Work out the finished part from the listing and answer in its coordinate system (mm). Face numbers are marked on the shaded views. A direction names the side the tool comes from. Coordinates: 2 decimals unless noted, no trailing zeros. Write each loop counter-clockwise with the first axis right and the second up, starting at its lowest first coordinate (ties: lowest second). Pieces come first, ordered by that corner, then holes. Notation, with made-up numbers: (-2.75, 16.5) - (24.25, 16.5) arc R13 cw to (24.25, 33.5) - close; hole circle Ø5 at (-3.5, -25). An arc over 180 degrees is marked (long way). One line per item, written item: value.
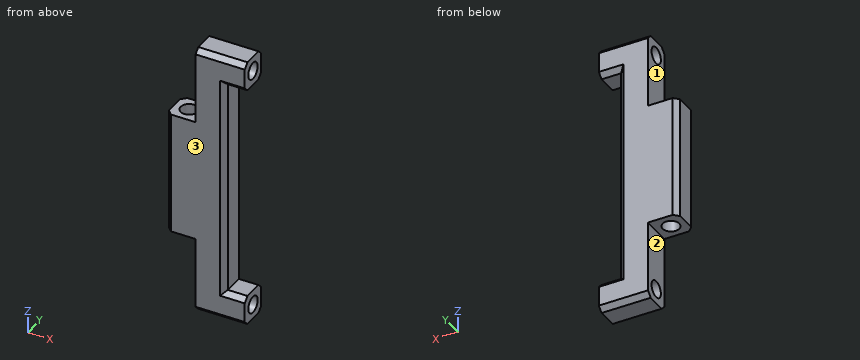
Autodesk Inventor part; units mm, degrees
ref_plane "YZ Plane" through (0, 0, 0) normal (1, 0, 0) x (0, 1, 0)
ref_plane "XZ Plane" through (0, 0, 0) normal (0, 1, 0) x (-1, 0, 0)
ref_plane "XY Plane" through (0, 0, 0) normal (0, 0, 1) x (1, 0, 0)
sketch "Sketch1" plane through (0, 0, 0) normal (0, 1, 0) x (-1, 0, 0)
  line L0 (0, 0) -> (0, -6)
  line L1 (0, -6) -> (4, -6)
  line L2 (4, -6) -> (4, -50)
  line L3 (4, -50) -> (0, -50)
  line L4 (0, -50) -> (0, -56)
  line L5 (0, -56) -> (10, -56)
  line L6 (0, 0) -> (10, 0)
  line L7 (10, 0) -> (10, -15.5)
  line L8 (10, -15.5) -> (16, -15.5)
  line L9 (16, -40.5) -> (10, -40.5)
  line L10 (10, -40.5) -> (10, -56)
  line L11 (16, -15.5) -> (16, -40.5)
  point P0 (0, -3)
  point P1 (0, -53)
  dimension "d0" = 25
  dimension "d1" = 6
  dimension "d2" = 50
  dimension "d3" = 6
  dimension "d4" = 4
  dimension "d17" = 6
extrude "Extrusion1" add sketch "Sketch1" along normal blind 6
sketch "Sketch2" plane through (0, 0, 0) normal (1, 0, 0) x (0, 0, -1)
  line L0 (15.5, 6) -> (0, 6)
  line L1 (6, 0) -> (50, 0)
  line L2 (0, 6) -> (6, 0) construction
  line L3 (50, 0) -> (56, 0)
  line L4 (50, 0) -> (56, 6) construction
  circle A0 centre (3, 3) radius 1.7
  circle A1 centre (53, 3) radius 1.7
  point P0 (0, 0)
  dimension "d8" = 3.4
extrude "Extrusion2" cut sketch "Sketch2" against normal through all
sketch "Sketch3" plane through (-16, 0, -15.5) normal (0, 0, 1) x (1, 0, 0)
  line L0 (16, 0) -> (6, 0)
  line L1 (0, 6) -> (6, 0) construction
  circle A0 centre (3, 3) radius 1.7
  dimension "d11" = 3.4
extrude "Extrusion3" cut sketch "Sketch3" against normal through all
chamfer "Chamfer1" distance 1 angle 45 12 edges at (-5, 6, 0) (-5, 0, 0) (-16, 6, -28) (-16, 0, -28) (-2, 6, -50) (-5, 6, -56) (-5, 0, -56) (-2, 0, -50) (-4, 6, -28) (-4, 0, -28) (-2, 6, -6) (-2, 0, -6)
equation "\"d3\" = d1"
equation "\"d6\" = d1"
properties part number "camadapter"
Item 1: Section A-A, the plane z = -3 is taken. Determine the outline of the cut face in (x, y), then the cut area to 3 significant figures.
Evaluation:
outline: (-10, 0) - (0, 0) - (0, 1.3) - (-10, 1.3) - close; (-10, 4.7) - (0, 4.7) - (0, 6) - (-10, 6) - close
area: 26.0 mm2
Item 2: Which of the six approach directions +Z, -Z, +X, -X, +Y, -Y give full straight-line access (tool end or side, diameter ignored) to the marked faces 1, 2 and 3?
Evaluation:
face 1: +Z, -X, +Y, -Y
face 2: -Z, -X, +Y, -Y
face 3: +Z, -Z, +X, -X, -Y
Item 3: Consider probe 1 along X at (y, z) = (2.85, -40); probe 2 along Z at (x, y) = (-1.5, 4.85); probe 3 along Y at (x, z) = (-13, -22.5). Determine where each line is inside the solid, lowest interval first.
Evaluation:
probe 1: x = -16 to -14.69, -11.31 to -4
probe 2: z = -56 to -50, -6 to 0
probe 3: y = 0 to 1.3, 4.7 to 6
Item 4: Section B-B, the plane x = -9.5 is taken. Determine the outline of the cut face in (y, z).
Evaluation:
outline: (0, -55) - (1, -56) - (5, -56) - (6, -55) - (6, -1) - (5, 0) - (1, 0) - (0, -1) - close; hole circle Ø3.4 at (3, -53); hole circle Ø3.4 at (3, -3)
Item 5: Section D-D, the plane x = -13 is taken. Determine the outline of the cut face in (y, z), then the cut area to 3 significant figures.
Evaluation:
outline: (0, -40.5) - (1.3, -40.5) - (1.3, -15.5) - (0, -15.5) - close; (4.7, -40.5) - (6, -40.5) - (6, -15.5) - (4.7, -15.5) - close
area: 65.0 mm2
Item 6: Section C-C, the plane y = 3 is taken. Determine the outline of the cut face in (x, z), then the cut area to 3 significant figures.
Evaluation:
outline: (-16, -40.5) - (-14.7, -40.5) - (-14.7, -15.5) - (-16, -15.5) - close; (-11.3, -40.5) - (-10, -40.5) - (-10, -51.3) - (0, -51.3) - (0, -50) - (-4, -50) - (-4, -6) - (0, -6) - (0, -4.7) - (-10, -4.7) - (-10, -15.5) - (-11.3, -15.5) - close; (-10, -56) - (0, -56) - (0, -54.7) - (-10, -54.7) - close; (-10, -1.3) - (0, -1.3) - (0, 0) - (-10, 0) - close
area: 381 mm2
Item 7: Given pin 1 (1.8 mm diameter, centred on y = 2.5, z = -48, fed in from -X); pin 2 (1.2 mm diameter, centred on y = 3.5, z = -34, fed in from +X), each flat-ended and moving along its own axis, determine where each tip first touches the part or whether it passes through.
Evaluation:
pin 1: stops at x = -10
pin 2: stops at x = -4
